```python
from build123d import *

# Parameters (mm, degrees)
F1_DEPTH = 6


with BuildPart() as f1:
    # F0 (on Top) → F1 (new body)
    with BuildSketch(Plane.XY):
        with BuildLine():
            ThreePointArc((-8.05516, 8.416466), (-8.132287, 8.238597), (-8.059079, 8.059079))
            Line((-8.059079, 8.059079), (-7.071068, 7.071068))
            ThreePointArc((-7.071068, 7.071068), (-4.316488, 9.020417), (-1.070361, 9.942551))
            Line((-1.070361, 9.942551), (-1.219918, 11.331783))
            ThreePointArc((-1.219918, 11.331783), (-1.313786, 11.501414), (-1.500685, 11.552941))
            ThreePointArc((-1.500685, 11.552941), (-5.028709, 10.508786), (-8.05516, 8.416466))
        make_face()
    extrude(amount=F1_DEPTH)


solid = f1.part
```
Could you check a few things on this model? Use its own coordinates, in mm. Coordinates: 2 decimals unless noted, no trailing zeros. Loops run counter-clockwise (first coordinate to the right, second up) from the corner with the lowest first, then second, coordinate; pieces in that order, holes last.
1) Please list where these lines run through material, in increasing order: line 1 along Y through (x, z) = (-6.25, 3.15); line 2 along X through (y, z) = (7.7, 2.2); line 3 along X through (y, z) = (8.5, 2.3).
Reported:
line 1: y = 7.81 to 9.83
line 2: x = -7.7 to -6.38
line 3: x = -7.97 to -5.27
2) Will this pin go through, and if not, where does the flat tip stop? pin 1 Ø1.5 at (y, z) = (8.5, 4) entering from +X.
Reported:
pin 1: stops at x = -3.8
3) Imagine slicing it at C-C (x = -2.5). List the corners of the cut face in (y, z) for me.
Reported:
outline: (9.68, 0) - (11.38, 0) - (11.38, 6) - (9.68, 6) - close
4) Imagine slicing it at B-B (y = 8.95). List the corners of the cut face in (x, z) for me.
Reported:
outline: (-7.46, 0) - (-4.46, 0) - (-4.46, 6) - (-7.46, 6) - close
5) Imagine slicing it at A-A (z = 0.65). List the corners of the cut face in (x, y) for me.
Reported:
outline: (-8.06, 8.06) - (-7.07, 7.07) arc R10 cw to (-1.07, 9.94) - (-1.22, 11.33) arc R0.25 ccw to (-1.5, 11.55) arc R11.65 ccw to (-8.06, 8.42) arc R0.25 ccw to start
